Here's how the part is built. I have some questions about the finished solid (model axes, mm). Face numbers are marked on the shaded views. A direction names the side the tool comes from. Round coordinates to 2 decimals unless told otherwise and drop trailing zeros. Loops run counter-clockwise (first coordinate to the right, second up) from the corner with the lowest first, then second, coordinate; pieces in that order, holes last. Notation, with made-up numbers: (65.5, 61) - (121.5, 61) arc R21 cw to (121.5, 71) - close; hole circle Ø11 at (-29, 51). An arc over 180 degrees is marked (long way). Answer as a JSON object with one key per item and string values. Group by question number.
1) If I drill on line 1 along X through (y, z) = (-4, 6.75); line 2 along Y through (x, z) = (-27, 9); line 3 along Y through (x, z) = (-25, 7), over which ranges is the centre line in solid material (lowest first)? Write a range as [from, to].
2) Which directions (+Z, -Z, +X, -X, +Y, -Y) give clear straight access to the entire face, cutting with the end or side of a thin tool? Please do the marked faces 1 and 2.
3) If we mould it in two halves opening along X, with no side actions, what happens to the marked faces 3, 4 and 5? For each: pulls with the +X half, pulls with the -X half, needs draft (parallel to the pull), parting line crosses it, or undercut.
4) I want a section at C-C, the plane x = 17.5. Please give me the cut outline in (y, z).
5) I want a section at B-B, the plane y = -5. Please give me the cut outline in (x, z).
6) Will these pins go through, and if not, where does the flat tip stop? P1, Ø2, axis at y = 22.5, z = 8.5, coming from the -X side; P2, Ø5, axis at x = -15, y = -8, coming from the -Z side.
7) I want a section at A-A, the plane z = 5. Please give me the cut outline in (x, y).
8) I want a section at D-D, the plane x = -25. Please give me the cut outline in (y, z).
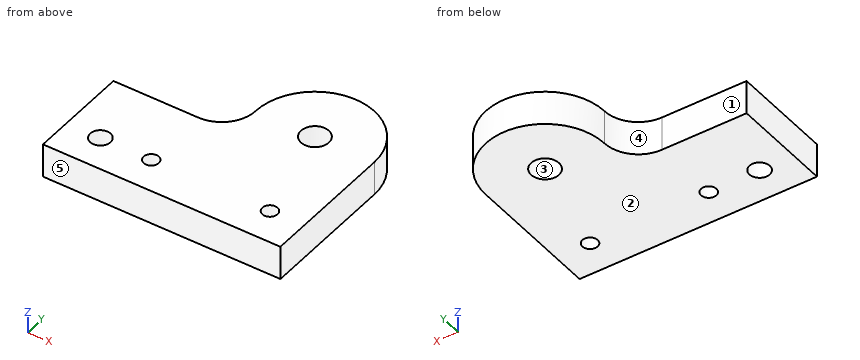
from build123d import *

# Parameters (mm, degrees)
SKETCH_2_R      = 4.1
SKETCH_2_R_2    = 3
SKETCH_2_R_3    = 2.25
EXTRUDE_1_DEPTH = 10


with BuildPart() as part:
    # 草图2 → 凸台-拉伸1 (new body)
    with BuildSketch(Plane.XY):
        with BuildLine():
            Line((-35, 15), (-10, 15))
            ThreePointArc((-10, 15), (-2.928932188, 17.928932188), (0, 25))
            ThreePointArc((0, 25), (17.5, 42.5), (35, 25))
            Line((35, 25), (35, 15))
            Line((35, 15), (35, -15))
            Line((35, -15), (-35, -15))
            Line((-35, -15), (-35, 15))
        make_face()
        with Locations((17.5, 25)):
            Circle(SKETCH_2_R, mode=Mode.SUBTRACT)
        with Locations((-25, -5)):
            Circle(SKETCH_2_R_2, mode=Mode.SUBTRACT)
        with Locations((-10, -5)):
            Circle(SKETCH_2_R_3, mode=Mode.SUBTRACT)
        with Locations((25, -5)):
            Circle(SKETCH_2_R_3, mode=Mode.SUBTRACT)
    extrude(amount=EXTRUDE_1_DEPTH)


solid = part.part
Outcome:
{
 "1": {"line 1": "[-35, -27.83], [-22.17, -12.02], [-7.98, 22.98], [27.02, 35]", "line 2": "[-15, -7.24], [-2.76, 15]", "line 3": "[-15, -8], [-2, 15]"},
 "2": {"face 1": "+Z, -Z, -X, +Y", "face 2": "-Z, +X, -X, +Y, -Y"},
 "3": {"face 3": "undercut", "face 4": "pulls with the -X half", "face 5": "needs draft"},
 "4": {"outline": "(-15, 0) - (20.9, 0) - (20.9, 10) - (-15, 10) - close; (29.1, 0) - (42.5, 0) - (42.5, 10) - (29.1, 10) - close"},
 "5": {"outline": "(-35, 0) - (-28, 0) - (-28, 10) - (-35, 10) - close; (-22, 0) - (-12.25, 0) - (-12.25, 10) - (-22, 10) - close; (-7.75, 0) - (22.75, 0) - (22.75, 10) - (-7.75, 10) - close; (27.25, 0) - (35, 0) - (35, 10) - (27.25, 10) - close"},
 "6": {"P1": "x = -0.63", "P2": "z = 0"},
 "7": {"outline": "(-35, -15) - (35, -15) - (35, 25) arc R17.5 ccw to (0, 25) arc R10 cw to (-10, 15) - (-35, 15) - close; hole circle Ø6 at (-25, -5); hole circle Ø4.5 at (-10, -5); hole circle Ø8.2 at (17.5, 25); hole circle Ø4.5 at (25, -5)"},
 "8": {"outline": "(-15, 0) - (-8, 0) - (-8, 10) - (-15, 10) - close; (-2, 0) - (15, 0) - (15, 10) - (-2, 10) - close"}
}
